```python
from build123d import *

# Parameters (mm, degrees)
EXTRUDE_THIN1_DEPTH = 4


with BuildPart() as part:
    # Sketch2 → Extrude-Thin1 (new body)
    with BuildSketch(Plane(origin=(0, 0, 0), x_dir=(1, 0, 0), z_dir=(0, 1, 0))):
        with BuildLine():
            Line((0, -6.5), (0, -0.503115295))
            ThreePointArc((0, -0.503115295), (0.029732441, -0.413473149), (0.107142857, -0.359368068))
            ThreePointArc((0.107142857, -0.359368068), (0.375, 0), (0.107142857, 0.359368068))
            ThreePointArc((0.107142857, 0.359368068), (0.029732441, 0.413473149), (0, 0.503115295))
            Line((0, 0.503115295), (0, 6.5))
            Line((0, 6.5), (0.12, 6.5))
            Line((0.12, 6.5), (0.12, 0.503115295))
            ThreePointArc((0.12, 0.503115295), (0.125946488, 0.485186866), (0.141428571, 0.47436585))
            ThreePointArc((0.141428571, 0.47436585), (0.495, 0), (0.141428571, -0.47436585))
            ThreePointArc((0.141428571, -0.47436585), (0.125946488, -0.485186866), (0.12, -0.503115295))
            Line((0.12, -0.503115295), (0.12, -6.5))
            Line((0.12, -6.5), (0, -6.5))
        make_face()
    extrude(amount=EXTRUDE_THIN1_DEPTH)


solid = part.part
```
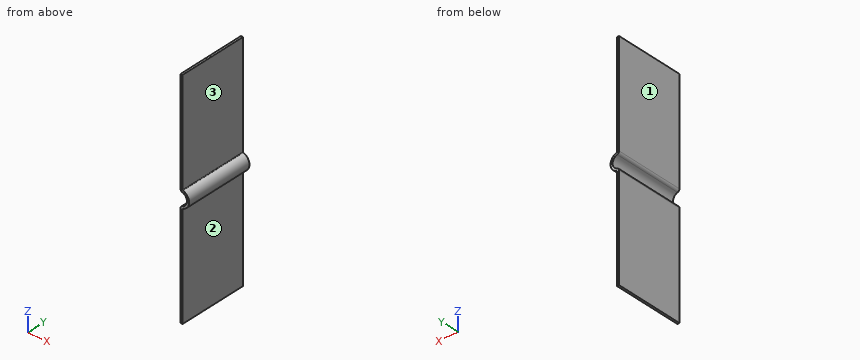
Geometry check sheet. Reference: the model listing, model coordinates, mm. Face numbers are marked on the shaded views. A direction names the side the tool comes from. Round coordinates to 2 decimals unless told otherwise and drop trailing zeros. Order: outer loops, then holes, each group sorted by start corner. A loop starts at its lowest first (then second) coordinate and runs counter-clockwise, first axis right, second up. Notation, with made-up numbers: (87.5, 77.25) -> (128.5, 77.25) arc R27 cw to (128.5, 96.25) -> close; hole circle Ø7 at (23, 10.5). An arc over 180 degrees is marked (long way). Return JSON: item names as keys, results as strings. Group by question number.
Q1. Section check C-C, the plane z = -5. Record the boundary of the cut face in (x, y).
Q2. Section check A-A, the plane x = 0.3. Record the boundary of the cut face in (y, z) (3 decimals), plus the area to 3 significant figures.
Q3. Section check B-B, the plane y = 1.85. Record the boundary of the cut face in (x, z) (3 decimals).
Q4. Gauge pin test, flat end, axial feed: pin 1 (1.2 mm diameter, centred on y = 1.5, z = 4, fed in from +X). Record the tip position at first contact, or that the pin passes through.
Q5. Tool access check on the marked faces 1, 2 and 3. Record the directions out of +Z, -Z, +X, -X, +Y, -Y that give a thin tool (end or side, any length) a straight path to the whole face; none if there is none.
Q6. Material ranges on probe 1 along Z at (x, y) = (0.3, 2.85) (3 decimals), recorded low to high. Write a range as from..to.
Numbers:
{
 "1": {"outline": "(0, 0) -> (0.12, 0) -> (0.12, 4) -> (0, 4) -> close"},
 "2": {"outline": "(0, -0.394) -> (4, -0.394) -> (4, -0.225) -> (0, -0.225) -> close; (0, 0.225) -> (4, 0.225) -> (4, 0.394) -> (0, 0.394) -> close", "area": "1.35 mm^2"},
 "3": {"outline": "(0, -6.5) -> (0.12, -6.5) -> (0.12, -0.503) arc R0.03 cw to (0.141, -0.474) arc R0.495 ccw to (0.141, 0.474) arc R0.03 cw to (0.12, 0.503) -> (0.12, 6.5) -> (0, 6.5) -> (0, 0.503) arc R0.15 ccw to (0.107, 0.359) arc R0.375 cw to (0.107, -0.359) arc R0.15 ccw to (0, -0.503) -> close"},
 "4": {"pin 1": "x = 0.12"},
 "5": {"face 1": "+Z, -Z, -X, +Y, -Y", "face 2": "-Z, +X, +Y, -Y", "face 3": "+Z, +X, +Y, -Y"},
 "6": {"probe 1": "-0.394..-0.225, 0.225..0.394"}
}
